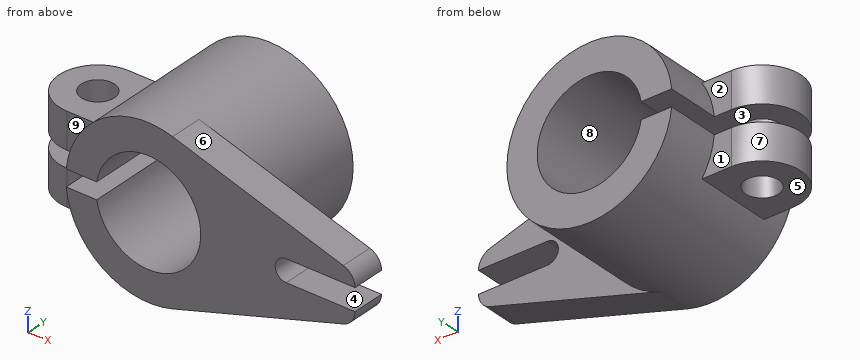
Autodesk Fusion 360 part; units mm, degrees
sketch "Sketch1" plane through (0, 0, 0) normal (0, 1, 0) x (1, 0, 0)
  circle A0 centre (0, 0) radius 19
  circle A1 centre (0, 0) radius 30
  line L0 (0, 0) -> (50, 0) construction
  line L1 (50, 0) -> (75, 0) construction
  line L2 (50, 4) -> (75, 4)
  line L3 (50, -4) -> (75, -4)
  line L4 (8.7717, 28.689) -> (70.7543, 9.7378)
  arc A2 (75, 4) -> (70.7543, 9.7378) centre (69, 4) ccw
  arc A3 (50, 4) -> (50, -4) centre (50, 0) ccw
  line L5 (8.7717, -28.689) -> (70.7543, -9.7378)
  arc A4 (70.7543, -9.7378) -> (75, -4) centre (69, -4) ccw
  dimension "d1" = 38
  dimension "d2" = 60
  dimension "d3" = 50
  dimension "d4" = 8
  dimension "d5" = 25
  dimension "d6" = 4
  dimension "d7" = 4
  dimension "d8" = 12
extrude "Extrude1" add sketch "Sketch1" along normal blind 44 contours A1
extrude "Extrude2" add sketch "Sketch1" along normal blind 12 contours A1 L2 L3 L4 A2 A3 L5 A4
sketch "Sketch2" plane through (0, 0, 0) normal (0, 0, 1) x (1, 0, 0)
  circle A0 centre (-36, 22) radius 6
  line L0 (-36, 36) -> (-22, 36)
  line L1 (-22, 36) -> (-22, 8)
  line L2 (-22, 8) -> (-36, 8)
  arc A1 (-36, 36) -> (-36, 8) centre (-36, 22) ccw
  line L3 (30, 0) -> (-30, 0)
  dimension "d14" = 28
  dimension "d15" = 12
  dimension "d16" = 8
  dimension "d17" = 36
extrude "Extrude3" add sketch "Sketch2" along normal mid plane 32
sketch "Sketch3" plane through (0, 44, 0) normal (0, 1, 0) x (-1, 0, 0)
  circle A0 centre (0, 0) radius 19
  circle A1 centre (0, 0) radius 30
  line L0 (54, -3) -> (11, -3)
  line L1 (11, -3) -> (11, 3)
  line L2 (11, 3) -> (54, 3)
  line L3 (54, 3) -> (54, -3)
  line L4 (0, 0) -> (-50, 0)
  dimension "d20" = 3
  dimension "d21" = 3
  dimension "d22" = 11
  dimension "d23" = 43
extrude "Extrude4" cut sketch "Sketch3" against normal up to surface (44 mm away) contours A0 A1 L0 L2 | A1 L0 L2 L3
extrude "Extrude5" add 1 faces at (26.2783, 44, 0) along direction (0, 1, 0) blind 11.305
ref_plane "WorkPlane1" through (41.8858, 85.34, 0) normal (0, 1, 0) x (1, 0, 0)
ref_plane "WorkPlane2" through (0, 0, 57.35) normal (0, 0, 1) x (1, 0, 0)
Can you work these out from the model? Positions are in its coordinate system, mm. Face numbers are marked on the shaded views. A direction names the side the tool comes from. Coordinates: 2 decimals unless noted, no trailing zeros. Loops run counter-clockwise (first coordinate to the right, second up) from the corner with the lowest first, then second, coordinate; pieces in that order, holes last.
1) For pin 1 (9.5 mm diameter, centred on x = -37.5, y = 25.5, fed in from -Z); pin 2 (1 mm diameter, centred on y = 19, z = 18.5, fed in from -X); pin 3 (12 mm diameter, centred on x = -27.5, y = 16.5, fed in from +Z), each with a flat end and sliding along its axis, tell me the tip position at first contact or that it passes through.
2) Imagine slicing it at B-B on z = 0. List the corners of the cut face in (x, y) for me (3 decimals), plus the area to 3 significant figures.
3) Which directions (+Z, -Z, +X, -X, +Y, -Y) give clear straight access to the entire face, cutting with the end or side of a thin tool? Please do the marked faces 1, 2, 3, 4 and 5.
4) I need wall thicknesses on probe 1 along Z at (x, y) = (0, 33); probe 2 along X at (y, z) = (22, 8.25); probe 3 along Y at (x, z) = (-36, 7). Which ranges of each line are inside material? Lowest first, please.
5) Thinking about a two-plate mould opening in X: for the marked faces 6, 7, 8 and 9, which applies, pulls with the +X half, pulls with the -X half, needs draft (parallel to the pull), parting line crosses it, or undercut?
6) Imagine slicing it at C-C on y = 4. List the corners of the cut face in (x, z) for me.
7) Imagine slicing it at A-A on x = 0. List the corners of the cut face in (y, z) for me (3 decimals), plus the area to 3 significant figures.
8) Imagine slicing it at D-D on x = 54. List the corners of the cut face in (y, z) for me, plus the area to 3 significant figures.
Completed:
1. pin 1: stops at z = -16
1. pin 2: stops at x = -24
1. pin 3: stops at z = 20.92
2. outline: (19, 0) - (46, 0) - (46, 12) - (30, 12) - (30, 55.305) - (19, 55.305) - close
2. area: 800 mm2
3. face 1: -Z, -X, +Y
3. face 2: +Z, -X, +Y
3. face 3: -X, +Y, -Y
3. face 4: +X, +Y, -Y
3. face 5: -Z, -X, +Y, -Y
4. probe 1: z = -30 to -19, 19 to 30
4. probe 2: x = -50 to -42, -30 to -17.12, 17.12 to 28.84
4. probe 3: y = 8 to 16, 28 to 36
5. face 6: pulls with the +X half
5. face 7: pulls with the -X half
5. face 8: undercut
5. face 9: needs draft
6. outline: (-29.85, -3) arc R30 ccw to (8.77, -28.69) - (70.75, -9.74) arc R6 ccw to (75, -4) - (50, -4) arc R4 cw to (50, 4) - (75, 4) arc R6 ccw to (70.75, 9.74) - (8.77, 28.69) arc R30 ccw to (-29.85, 3) - (-18.76, 3) arc R19 cw (long way) to (-18.76, -3) - close
7. outline: (0, -30) - (55.305, -30) - (55.305, -19) - (0, -19) - close; (0, 19) - (55.305, 19) - (55.305, 30) - (0, 30) - close
7. area: 1,220 mm2
8. outline: (0, -14.86) - (12, -14.86) - (12, -4) - (0, -4) - close; (0, 4) - (12, 4) - (12, 14.86) - (0, 14.86) - close
8. area: 261 mm2
